Design review of the part built by this model. Coordinates are the model's own, in mm. Face numbers are marked on the shaded views. A direction names the side the tool comes from. Coordinates: 2 decimals unless noted, no trailing zeros. Write each loop counter-clockwise with the first axis right and the second up, starting at its lowest first coordinate (ties: lowest second). Pieces come first, ordered by that corner, then holes.
Q1. Take a section at D-D (z = 6.5). Give the boundary of the cut face in (x, y).
Q2. Take a section at C-C (z = 30). Give the boundary of the cut face in (x, y), and give its area (3 significant figures).
Q3. Mouldability with a two-part tool opening along Y and no side actions: class the marked faces 1, 2 and 3 as pulls with the +Y half, pulls with the -Y half, needs draft (parallel to the pull), parting line crosses it, or undercut.
Q4. Take a section at A-A (x = 25.4). Give the boundary of the cut face in (y, z).
Q5. Take a section at B-B (x = -24). Give the boundary of the cut face in (y, z).
Q6. Machinability: for the marked faces 4, 5, 6 and 7, which of the approach directions +Z, -Z, +X, -X, +Y, -Y give a long, thin tool a straight path to every point of the face, cutting with its end or side? Answer none if there is none.
Q7. For probe 1 along Y at (x, z) = (14.5, 4.5); probe 2 along Z at (x, y) = (25.4, 41.5); probe 3 along Y at (x, z) = (54, 2), list the stretches that pass through material, from the lowest coordinate up.
Q8. Insertion check: pin 1 (12 mm diameter, centred on x = 26.5, y = -40.5, fed in from -Z); pin 2 (20 mm diameter, centred on x = 25.4, z = 22.225, fed in from +Y); pin 3 (1.5 mm diameter, centred on y = 5, z = 34, fed in from +X); pin 4 (1.3 mm diameter, centred on y = 12.5, z = 20.5, fed in from +X). Each pin has a flat end and moves straight along its axis. Give the tip position at first contact, or say it passes through.
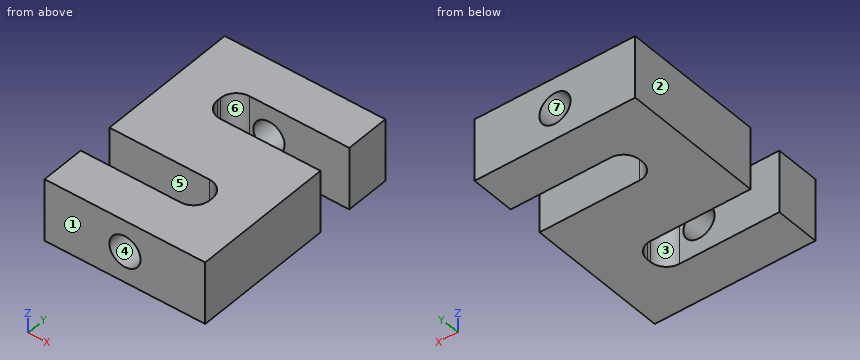
```python
from build123d import *

# Parameters (mm, degrees)
BOSS_EXTRUDE1_DEPTH      = 44.45
FILLET1_R                = 11.43
F_1_8_TAPPED_HOLE1_D     = 22.225
F_1_8_TAPPED_HOLE1_DEPTH = 31.75
F_1_8_TAPPED_HOLE2_D     = 22.225
F_1_8_TAPPED_HOLE2_DEPTH = 31.75


with BuildPart() as part:
    # Sketch1 → Boss-Extrude1 (new body)
    with BuildSketch(Plane.XY):
        Polygon((82.55, 0), (0, 0), (0, 25.4), (82.55, 25.4), (82.55, 57.15), (-31.75, 57.15), (-31.75, -44.45), (50.8, -44.45), (50.8, -69.85), (-31.75, -69.85), (-31.75, -101.6), (82.55, -101.6), align=None)
    extrude(amount=BOSS_EXTRUDE1_DEPTH)

    # Fillet1
    fillet1_edges = [part.edges().sort_by_distance(p)[0] for p in [
        (50.8, -69.85, 22.225),
        (50.8, -44.45, 22.225),
        (0, 25.4, 22.225),
        (0, 0, 22.225),
    ]]
    fillet(fillet1_edges, radius=FILLET1_R)

    # 1-8 Tapped Hole1
    with Locations(Plane.XZ.offset(101.6)):
        with Locations((25.4, 22.225)):
            Hole(F_1_8_TAPPED_HOLE1_D / 2, depth=F_1_8_TAPPED_HOLE1_DEPTH)

    # 1-8 Tapped Hole2
    with Locations(Plane(origin=(0, 57.15, 0), x_dir=(-1, 0, 0), z_dir=(0, 1, 0))):
        with Locations((-25.4, 22.225)):
            Hole(F_1_8_TAPPED_HOLE2_D / 2, depth=F_1_8_TAPPED_HOLE2_DEPTH)


solid = part.part
```
Response:
1. outline: (-31.75, -101.6) - (82.55, -101.6) - (82.55, 0) - (11.43, 0) arc R11.43 cw to (0, 11.43) - (0, 13.97) arc R11.43 cw to (11.43, 25.4) - (82.55, 25.4) - (82.55, 57.15) - (-31.75, 57.15) - (-31.75, -44.45) - (39.37, -44.45) arc R11.43 cw to (50.8, -55.88) - (50.8, -58.42) arc R11.43 cw to (39.37, -69.85) - (-31.75, -69.85) - close
2. outline: (-31.75, -101.6) - (17.46, -101.6) - (17.46, -69.85) - (-31.75, -69.85) - close; (-31.75, -44.45) - (39.37, -44.45) arc R11.43 cw to (50.8, -55.88) - (50.8, -58.42) arc R11.43 cw to (39.37, -69.85) - (33.34, -69.85) - (33.34, -101.6) - (82.55, -101.6) - (82.55, 0) - (11.43, 0) arc R11.43 cw to (0, 11.43) - (0, 13.97) arc R11.43 cw to (11.43, 25.4) - (17.46, 25.4) - (17.46, 57.15) - (-31.75, 57.15) - close; (33.34, 25.4) - (82.55, 25.4) - (82.55, 57.15) - (33.34, 57.15) - close
2. area: 13,100 mm2
3. face 1: pulls with the -Y half
3. face 2: needs draft
3. face 3: undercut
4. outline: (-101.6, 0) - (-69.85, 0) - (-69.85, 11.11) - (-101.6, 11.11) - close; (-101.6, 33.34) - (-69.85, 33.34) - (-69.85, 44.45) - (-101.6, 44.45) - close; (-44.45, 0) - (0, 0) - (0, 44.45) - (-44.45, 44.45) - close; (25.4, 0) - (57.15, 0) - (57.15, 11.11) - (25.4, 11.11) - close; (25.4, 33.34) - (57.15, 33.34) - (57.15, 44.45) - (25.4, 44.45) - close
5. outline: (-101.6, 0) - (-69.85, 0) - (-69.85, 44.45) - (-101.6, 44.45) - close; (-44.45, 0) - (57.15, 0) - (57.15, 44.45) - (-44.45, 44.45) - close
6. face 4: -Y
6. face 5: +Z, -Z, -X
6. face 6: +Z, -Z, +X
6. face 7: +Y
7. probe 1: y = -101.6 to -69.85, -44.45 to 0, 25.4 to 57.15
7. probe 2: z = 0 to 11.11, 33.34 to 44.45
7. probe 3: y = -101.6 to 0, 25.4 to 57.15
8. pin 1: stops at z = 0
8. pin 2: stops at y = 0
8. pin 3: stops at x = 2.54
8. pin 4: stops at x = 0
